```python
from build123d import *

# Parameters (mm, degrees)
SKETCH1_W           = 23
SKETCH1_H           = 28
BOSS_EXTRUDE1_DEPTH = 75
BOSS_EXTRUDE2_DEPTH = 1.5
CUT_EXTRUDE1_DEPTH  = 87.521673585
FILLET1_R           = 1
SKETCH7_W           = 2
SKETCH7_H           = 7
CUT_EXTRUDE2_DEPTH  = 87.521673672
SKETCH8_W           = 31
SKETCH8_H           = 7
CUT_EXTRUDE3_DEPTH  = 0.5
FILLET2_SIZE        = 2.5
FILLET2_SIZE_2      = 4
FILLET3_R           = 2


with BuildPart() as part:
    # Sketch1 → Boss-Extrude1 (new body)
    with BuildSketch(Plane(origin=(0, 0, 0), x_dir=(1, 0, 0), z_dir=(0, 1, 0))):
        with BuildLine():
            Line((0, 0), (30, 0))
            Line((30, 0), (30, 31))
            Line((30, 31), (0, 31))
            Line((0, 31), (0, 25.798058069))
            ThreePointArc((0, 25.798058069), (3.5, 15.5), (0, 5.201941931))
            Line((0, 5.201941931), (0, 0))
        make_face()
        with Locations((17, 15.5)):
            Rectangle(SKETCH1_W, SKETCH1_H, mode=Mode.SUBTRACT)
    extrude(amount=BOSS_EXTRUDE1_DEPTH)

    # Sketch2 → Boss-Extrude2 (add)
    with BuildSketch(Plane.XZ):
        with BuildLine():
            Line((0, -25.798058069), (0, -31))
            Line((0, -31), (30, -31))
            Line((30, -31), (30, 0))
            Line((30, 0), (0, 0))
            Line((0, 0), (0, -5.201941931))
            ThreePointArc((0, -5.201941931), (3.55300213, -15.5), (0, -25.798058069))
        make_face()
    extrude(amount=BOSS_EXTRUDE2_DEPTH)

    # Sketch6 → Cut-Extrude1 (cut, through all)
    with BuildSketch(Plane.XY):
        Polygon((5.5, 75), (30, 43.5), (30, 75), align=None)
    extrude(amount=-CUT_EXTRUDE1_DEPTH, mode=Mode.SUBTRACT)

    # Fillet1
    fillet1_edges = [part.edges().sort_by_distance(p)[0] for p in [
        (0, 36.75, -31),
        (0, 36.75, 0),
        (0, 75, -28.399029035),
        (3.5, 75, -15.5),
        (0, -1.5, -2.600970965),
        (3.55300213, -1.5, -15.5),
        (0, -1.5, -28.399029035),
        (15, -1.5, -31),
        (30, -1.5, -15.5),
        (15, -1.5, 0),
        (0, 75, -2.600970965),
        (30, 21, -31),
        (2.75, 75, -31),
        (30, 21, 0),
        (17.75, 59.25, -31),
        (30, 43.5, -15.5),
        (17.75, 59.25, 0),
        (2.75, 75, 0),
    ]]
    fillet(fillet1_edges, radius=FILLET1_R)

    # Sketch7 → Cut-Extrude2 (cut, through all)
    with BuildSketch(Plane.XY):
        with Locations((6.5, 55)):
            Rectangle(SKETCH7_W, SKETCH7_H)
        with Locations((6.5, 10)):
            Rectangle(SKETCH7_W, SKETCH7_H)
    extrude(amount=-CUT_EXTRUDE2_DEPTH, mode=Mode.SUBTRACT)

    # Sketch8 → Cut-Extrude3 (cut)
    with BuildSketch(Plane(origin=(5.5, 0, 0), x_dir=(0, 0, -1), z_dir=(1, 0, 0))):
        with Locations((15.5, 55)):
            Rectangle(SKETCH8_W, SKETCH8_H)
        with Locations((15.5, 10)):
            Rectangle(SKETCH8_W, SKETCH8_H)
    extrude(amount=-CUT_EXTRUDE3_DEPTH, mode=Mode.SUBTRACT)

    # Fillet2
    # an asymmetric fillet: 4, 2.5 mm, written as the material it takes off along each edge
    with BuildSketch(Plane(origin=(5, 6.5, -31), x_dir=(-1, 0, 0), z_dir=(0, 1, 0)), Plane(origin=(5, 13.5, 0), x_dir=(-1, 0, 0), z_dir=(0, -1, 0))) as fillet2_piece_1:
        with BuildLine():
            Bezier((FILLET2_SIZE, 0), (0, 0), (0, FILLET2_SIZE_2), weights=[1, 0.707106781, 1])
            Line((0, FILLET2_SIZE_2), (0, 0))
            Line((0, 0), (FILLET2_SIZE, 0))
        make_face()
    extrude(amount=7, mode=Mode.SUBTRACT)
    with BuildSketch(Plane(origin=(5, 58.5, -31), x_dir=(-1, 0, 0), z_dir=(0, -1, 0)), Plane(origin=(5, 51.5, 0), x_dir=(-1, 0, 0), z_dir=(0, 1, 0))) as fillet2_piece_2:
        with BuildLine():
            Bezier((FILLET2_SIZE, 0), (0, 0), (0, -FILLET2_SIZE_2), weights=[1, 0.707106781, 1])
            Line((0, -FILLET2_SIZE_2), (0, 0))
            Line((0, 0), (FILLET2_SIZE, 0))
        make_face()
    extrude(amount=7, mode=Mode.SUBTRACT)

    # Fillet3
    fillet3_edges = [part.edges().sort_by_distance(p)[0] for p in [
        (5.5, 32.5, -29.5),
        (5.5, 3.25, -29.5),
        (5.5, 32.5, -1.5),
        (5.5, 3.25, -1.5),
        (5.5, 0, -15.5),
        (5.5, 66.75, -29.5),
        (17, 0, -1.5),
        (5.5, 66.75, -1.5),
        (28.5, 0, -15.5),
        (17, 0, -29.5),
        (28.5, 22.714285714, -29.5),
        (28.5, 22.714285714, -1.5),
    ]]
    fillet(fillet3_edges, radius=FILLET3_R)


solid = part.part
```
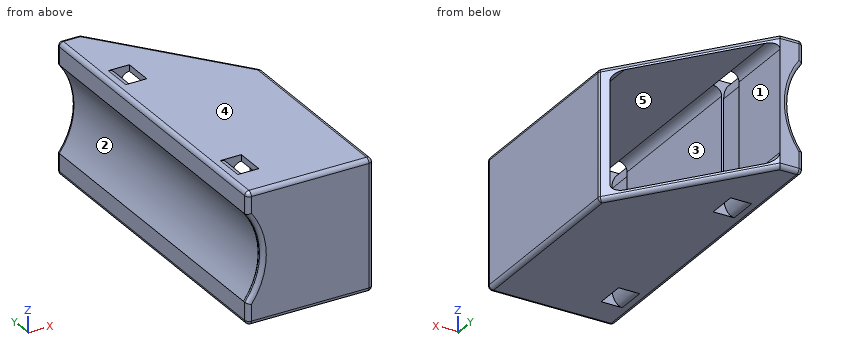
Could you check a few things on this model? Use its own coordinates, in mm. Face numbers are marked on the shaded views. A direction names the side the tool comes from. Coordinates: 2 decimals unless noted, no trailing zeros. Loops run counter-clockwise (first coordinate to the right, second up) from the corner with the lowest first, then second, coordinate; pieces in that order, holes last.
1) Imagine slicing it at A-A (y = 20.5). List the corners of the cut face in (x, z) for me.
Reported:
outline: (0, -30) arc R1 ccw to (1, -31) - (29, -31) arc R1 ccw to (30, -30) - (30, -1) arc R1 ccw to (29, 0) - (1, 0) arc R1 ccw to (0, -1) - (0, -5.2) arc R16.9 cw to (0, -25.8) - close; hole (5.5, -27.5) arc R2 ccw to (7.5, -29.5) - (26.5, -29.5) arc R2 ccw to (28.5, -27.5) - (28.5, -3.5) arc R2 ccw to (26.5, -1.5) - (7.5, -1.5) arc R2 ccw to (5.5, -3.5) - close
2) Which directions (+Z, -Z, +X, -X, +Y, -Y) give clear straight access to the entire face, cutting with the end or side of a thin tool? Please do the marked faces 4 and 5.
Reported:
face 4: +Z, +X, -X, +Y, -Y
face 5: +Y
3) Imagine slicing it at B-B (y = 53.5). State how many separate pieces and enclosed holes the cut face has, and give its area (3 significant figures).
Reported:
separate pieces: 3
enclosed holes: 0
area: 145 mm2
4) Please list where these lines run through material, in increasing order: line 1 along Z through (x, y) = (9.5, 53.5); line 2 along X through (y, z) = (32.5, -27); line 3 along X through (y, z) = (60, -4.5).
Reported:
line 1: z = -31 to -29.5, -1.5 to 0
line 2: x = 0 to 5.5, 28.5 to 30
line 3: x = 0 to 5.5
5) Thinking about a two-plate mould opening in X: for the marked faces 1, 2 and 3, which applies, released by +X, released by -X, zero draft, split by the parting line, or undercut?
Reported:
face 1: released by +X
face 2: released by -X
face 3: undercut
6) Will these pins go through, and if not, where does the flat tip stop? pin 1 Ø6 at (x, z) = (13, -23) entering from +Y; pin 2 Ø10 at (x, y) = (9.5, 57) entering from +Z; pin 3 Ø4 at (y, z) = (58.5, -25.5) entering from +X; pin 4 Ø5 at (y, z) = (19.5, -13.5) entering from -X.
Reported:
pin 1: stops at y = 0
pin 2: stops at z = 0
pin 3: stops at x = 5.5
pin 4: stops at x = 2.89
